Can you work these out from the model? Positions are in its coordinate system, mm. Give positions to 0.01 mm unless a question says otherwise; leave off trailing zeros. Order: outer loops, then holes, each group sorted by start corner. A loop starts at its lowest first (then second) coordinate and runs counter-clockwise, first axis right, second up. Notation, with made-up numbers: M -24.5,-8 L 10.5,-8 A17 cw 10.5,23 Z; hole C -28.75,61.5 d4. An arc over 180 degrees is marked long. Use one line per item in the form item = value. Start each with the question number.
1. I want a section at C-C, the plane x = 25.5. List the corners of the cut face in (y, z) for me, and give its area (3 significant figures).
2. I need wall thicknesses on L1, parallel to Y at x = -13, z = 0.75; L2, parallel to X at y = -8.5, z = 0.9; L3, parallel to X at y = -19, z = 1.55. Which ranges of each line are inside material? Lowest first, please.
3. I want a section at B-B, the plane y = 20. List the corners of the cut face in (x, z) for me.
4. Will these pins go through, and if not, where does the flat tip stop? P1, Ø1.5, axis at x = -3.5, z = 2.5, coming from the +Y side; P2, Ø1.5, axis at y = 7, z = 2.5, coming from the +X side; P3, Ø1.5, axis at x = 3, z = 0.5, coming from the -Y side.
5. I want a section at A-A, the plane z = 2.35. List the corners of the cut face in (x, y) for me.
Autodesk Fusion 360 part; units mm, degrees
sketch "Sketch1" plane through (0, 0, 0) normal (0, 0, 1) x (1, 0, 0)
  line L0 (13.5687, 24.844) -> (-12.9876, 25.1527)
  line L1 (-14.7311, 24.1729) -> (-28.2766, 1.3288)
  line L2 (-28.2999, -0.6711) -> (-15.2891, -23.8239)
  line L3 (-13.5687, -24.844) -> (12.9876, -25.1527)
  line L4 (14.7311, -24.1729) -> (28.2766, -1.3288)
  line L5 (28.2999, 0.6711) -> (15.2891, 23.8239)
  arc A0 (-12.9876, 25.1527) -> (-14.7311, 24.1729) centre (-13.0108, 23.1528) ccw
  arc A1 (15.2891, 23.8239) -> (13.5687, 24.844) centre (13.5455, 22.8441) ccw
  arc A2 (28.2766, -1.3288) -> (28.2999, 0.6711) centre (26.5563, -0.3087) ccw
  arc A3 (12.9876, -25.1527) -> (14.7311, -24.1729) centre (13.0108, -23.1528) ccw
  arc A4 (-15.2891, -23.8239) -> (-13.5687, -24.844) centre (-13.5455, -22.8441) ccw
  arc A5 (-28.2766, 1.3288) -> (-28.2999, -0.6711) centre (-26.5563, 0.3087) ccw
  point P0 (-12.5, 7.2169)
  dimension "d1" = 25
  dimension "d7" = 2
  dimension "d8" = 2
  dimension "d9" = 2
  dimension "d10" = 2
  dimension "d11" = 2
  dimension "d12" = 2
extrude "Extrude1" add sketch "Sketch1" along normal blind 3
Check result:
q1.outline = M -6.01,0 L 5.65,0 L 5.65,3 L -6.01,3 Z
q1.area = 35.0 mm2
q2.L1 = -24.85 to 25.15
q2.L2 = -23.9 to 24.02
q2.L3 = -18 to 17.8
q3.outline = M -17.21,0 L 17.44,0 L 17.44,3 L -17.21,3 Z
q4.P1 = 25.05
q4.P2 = 25.16
q4.P3 = -25.05
q5.outline = M -28.3,-0.67 L -15.29,-23.82 A2 ccw -13.57,-24.84 L 12.99,-25.15 A2 ccw 14.73,-24.17 L 28.28,-1.33 A2 ccw 28.3,0.67 L 15.29,23.82 A2 ccw 13.57,24.84 L -12.99,25.15 A2 ccw -14.73,24.17 L -28.28,1.33 A2 ccw Z
